Read the model definition and answer for the solid it produces. Units are mm, in the model's axes. Face numbers are marked on the shaded views. A direction names the side the tool comes from. Round coordinates to 2 decimals unless told otherwise and drop trailing zeros. Loops run counter-clockwise (first coordinate to the right, second up) from the corner with the lowest first, then second, coordinate; pieces in that order, holes last. Notation, with made-up numbers: M 85,-25 L 96,-25 A29 ccw 96,9 Z; hole C -5,-9.75 d10. An arc over 180 degrees is marked long. Write each question's results on one line, items separated by ' | '.
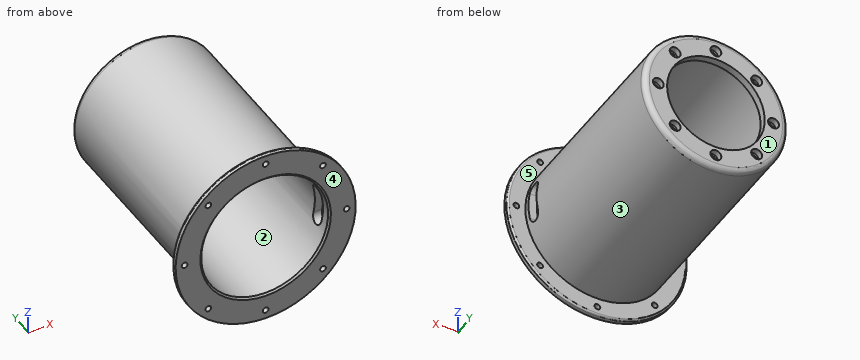
from build123d import *

# Parameters (mm, degrees)
SKETCH_1_R               = 40
EXTRUDE_1_DEPTH          = 120
SKETCH_2_R               = 35.25
CUT_EXTRUDE_1_DEPTH      = 115
SKETCH_3_R               = 27.1
CUT_EXTRUDE_2_DEPTH      = 133.664991614
PATTERN_CIRCULAR_1_COUNT = 8
SKETCH_7_R               = 50
SKETCH_7_R_2             = 40
EXTRUDE_2_DEPTH          = 3
SKETCH_8_R               = 1.6
CUT_EXTRUDE_3_DEPTH      = 137.707717412
PATTERN_CIRCULAR_2_COUNT = 8
FILLET_1_R               = 3
CHAMFER_1_SIZE           = 1
FILLET_2_R               = 1
CUT_EXTRUDE_4_DEPTH      = 159.11388304


with BuildPart() as part:
    # 草图1 → 凸台-拉伸1 (new body)
    with BuildSketch(Plane(origin=(0, 0, 0), x_dir=(1, 0, 0), z_dir=(0, 1, 0))):
        with Locations(Location((0, 0, 0), (0, 0, 270))):
            Circle(SKETCH_1_R)
    extrude(amount=EXTRUDE_1_DEPTH)

    # 草图2 → 切除-拉伸1 (cut)
    with BuildSketch(Plane.XZ):
        with Locations(Location((0, 0, 0), (0, 0, 270))):
            Circle(SKETCH_2_R)
    extrude(amount=-CUT_EXTRUDE_1_DEPTH, mode=Mode.SUBTRACT)

    # 草图3 → 切除-拉伸2 (cut, through all)
    with BuildSketch(Plane(origin=(0, 120, 0), x_dir=(1, 0, 0), z_dir=(0, 1, 0))):
        with Locations(Location((0, 0, 0), (0, 0, 270))):
            Circle(SKETCH_3_R)
    extrude(amount=-CUT_EXTRUDE_2_DEPTH, mode=Mode.SUBTRACT)

    # 草图6 → 打孔尺寸(%根据)内六角圆柱头螺钉的类型1 (revolve, cut)
    with BuildSketch(Plane(origin=(0, 120, -32), x_dir=(0, 0, 1), z_dir=(1, 0, 0))):
        Polygon((0, 0), (0, 120), (1.7, 120), (1.7, 3.4), (3, 3.4), (3, 0.025), (3.025, 0), align=None)
    hole_wizard_1 = revolve(axis=Axis((0, 126.35, -32), (0, -1, 0)), mode=Mode.SUBTRACT)

    # 阵列(圆周)1: 打孔尺寸(%根据)内六角圆柱头螺钉的类型1 ×8 about axis
    pattern_circular_1_axis = Axis((0, 0, 0), (0, 1, 0))
    for i in range(1, PATTERN_CIRCULAR_1_COUNT):
        add(hole_wizard_1.rotate(pattern_circular_1_axis, i * 360 / PATTERN_CIRCULAR_1_COUNT), mode=Mode.SUBTRACT)

    # 草图7 → 凸台-拉伸2 (add)
    with BuildSketch(Plane.XZ):
        with Locations(Location((0, 0, 0), (0, 0, 270))):
            Circle(SKETCH_7_R)
        with Locations(Location((0, 0, 0), (0, 0, 270))):
            Circle(SKETCH_7_R_2, mode=Mode.SUBTRACT)
    extrude(amount=-EXTRUDE_2_DEPTH)

    # 草图8 → 切除-拉伸3 (cut, through all)
    with BuildSketch(Plane(origin=(0, 3, 0), x_dir=(1, 0, 0), z_dir=(0, 1, 0))):
        with Locations(Location((0, -45, 0), (0, 0, 270))):
            Circle(SKETCH_8_R)
    cut_extrude_3 = extrude(amount=-CUT_EXTRUDE_3_DEPTH, mode=Mode.SUBTRACT)

    # 阵列(圆周)2: 切除-拉伸3 ×8 about axis
    pattern_circular_2_axis = Axis((0, 0, 0), (0, 1, 0))
    for i in range(1, PATTERN_CIRCULAR_2_COUNT):
        add(cut_extrude_3.rotate(pattern_circular_2_axis, i * 360 / PATTERN_CIRCULAR_2_COUNT), mode=Mode.SUBTRACT)

    # 圆角1
    fillet_1_edges = [part.edges().sort_by_distance(p)[0] for p in [
        (0, 120, -40),
    ]]
    fillet(fillet_1_edges, radius=FILLET_1_R)

    # 倒角1
    chamfer_1_edges = [part.edges().sort_by_distance(p)[0] for p in [
        (0, 115, -27.1),
        (0, 0, 35.25),
    ]]
    chamfer(chamfer_1_edges, length=CHAMFER_1_SIZE)

    # 圆角2
    fillet_2_edges = [part.edges().sort_by_distance(p)[0] for p in [
        (0, 3, 50),
    ]]
    fillet(fillet_2_edges, radius=FILLET_2_R)

    # 草图9 → 切除-拉伸4 (cut, through all)
    with BuildSketch(Plane(origin=(40, 0, 0), x_dir=(0, 0, -1), z_dir=(1, 0, 0))):
        with BuildLine():
            Line((-7.5, 14), (7.5, 14))
            ThreePointArc((7.5, 14), (11.5, 10), (7.5, 6))
            Line((7.5, 6), (-7.5, 6))
            ThreePointArc((-7.5, 6), (-11.5, 10), (-7.5, 14))
        make_face()
    extrude(amount=-CUT_EXTRUDE_4_DEPTH, mode=Mode.SUBTRACT)


solid = part.part
Item 1: The part is cut by section A-A (y = 11). Determine the outline of the cut face in (x, z), plus the area to 3 significant figures.
Outcome:
outline: M -38.35,-11.37 A40 ccw 38.35,-11.37 L 33.36,-11.37 A35.25 cw -33.36,-11.37 Z; M -38.35,11.37 L -33.36,11.37 A35.25 cw 33.36,11.37 L 38.35,11.37 A40 ccw Z | area: 903 mm2
Item 2: The part is cut by section B-B (y = 78). Determine the outline of the cut face in (x, z), plus the area to 3 significant figures.
Outcome:
outline: C 0,0 d80; hole C 0,0 d70.5 | area: 1,120 mm2
Item 3: Straight lines are drawn through the part: line 1 (Z direction, x = 9.5, y = 69.5); line 2 (Y direction, x = -33.5, z = 25.5); line 3 (X direction, y = 69.5, z = -6). For each, find the intervals that lie inside material, in ascending order.
Outcome:
line 1: z = -38.86 to -33.95, 33.95 to 38.86 | line 2: y = 0 to 3 | line 3: x = -39.55 to -34.74, 34.74 to 39.55
Item 4: The mould has two halves that part along Z. Classify the marked faces 1, 2 and 3: pulls with the +Z half, pulls with the -Z half, needs draft (parallel to the pull), parting line crosses it, or undercut.
Outcome:
face 1: needs draft | face 2: undercut | face 3: parting line crosses it
Item 5: Flat-ended cylindrical pins translate along their axes: pin 1 (8 mm diameter, centred on x = -37.5, z = -12, fed in from -Y); pin 2 (7 mm diameter, centred on x = 0, z = -32, fed in from -Y); pin 3 (1.9 mm diameter, centred on x = 31.82, z = -31.82, fed in from +Y); pin 4 (3.5 mm diameter, centred on x = 22.63, z = -22.63, fed in from -Y). Find the tip coordinate at first contact, or state that the pin passes through.
Outcome:
pin 1: stops at y = 0 | pin 2: stops at y = 0.75 | pin 3: passes through | pin 4: stops at y = 115
Item 6: The part is cut by section C-C (z = 0). State how many separate pieces and enclosed holes the cut face has, plus the area to 3 significant figures.
Outcome:
separate pieces: 8 | enclosed holes: 0 | area: 1,130 mm2
Item 7: For the marked faces 4 and 5, determine the directions among +Z, -Z, +X, -X, +Y, -Y from which every point of the face is accessible in a straight line to the end or side of a thin tool.
Outcome:
face 4: +Z, -Z, +X, -X, -Y | face 5: +Y
